Part model, mm, in its own coordinate system. Face numbers are marked on the shaded views. Round coordinates to 2 decimals unless told otherwise and drop trailing zeros. Loops run counter-clockwise (first coordinate to the right, second up) from the corner with the lowest first, then second, coordinate; pieces in that order, holes last. Notation, with made-up numbers: (84, 74) - (104, 74) arc R30 ccw to (104, 109) - close; hole circle Ø4 at (-35.75, 9). An arc over 180 degrees is marked (long way). Put each result on its own line as item: value.
from build123d import *

# Parameters (mm, degrees)
SKETCH1_R               = 9
SKETCH1_R_2             = 8.75
BOSS_EXTRUDE1_DEPTH     = 125
SKETCH2_R               = 2
CUT_EXTRUDE1_DEPTH      = 10
CUT_EXTRUDE1_DEPTH_BACK = 10


with BuildPart() as part:
    # Sketch1 → Boss-Extrude1 (new body)
    with BuildSketch(Plane(origin=(0, 0, 0), x_dir=(1, 0, 0), z_dir=(0, 1, 0))):
        Circle(SKETCH1_R)
        Circle(SKETCH1_R_2, mode=Mode.SUBTRACT)
    extrude(amount=BOSS_EXTRUDE1_DEPTH)

    # Sketch2 → Cut-Extrude1 (cut, two sides)
    with BuildSketch(Plane.XY) as cut_extrude1_sk:
        with Locations((0, 95)):
            Circle(SKETCH2_R)
        with Locations((0, 115)):
            Circle(SKETCH2_R)
        with Locations((0, 10)):
            Circle(SKETCH2_R)
    extrude(amount=CUT_EXTRUDE1_DEPTH, mode=Mode.SUBTRACT)
    extrude(cut_extrude1_sk.sketch, amount=-CUT_EXTRUDE1_DEPTH_BACK, mode=Mode.SUBTRACT)


solid = part.part
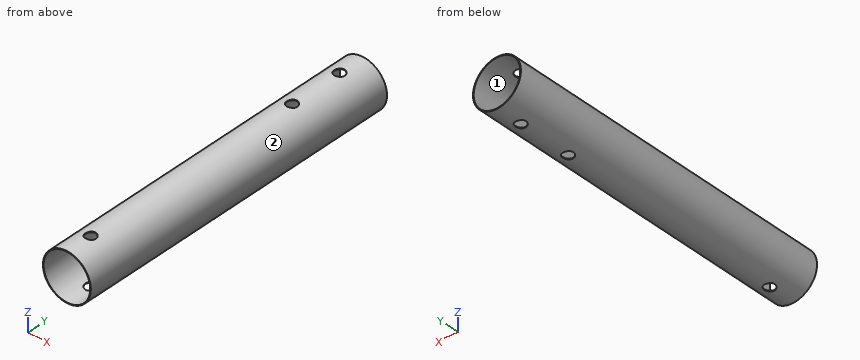
1. Band-saw the part on D-D (y = 73.5). List the corners of the cut face in (x, z).
A:
outline: circle Ø18 at (0, 0); hole circle Ø17.5 at (0, 0)
2. Two-plate mould, pull along Z, no slides. Class the marked faces 1 and 2: pulls with the +Z half, pulls with the -Z half, needs draft (parallel to the pull), parting line crosses it, or undercut.
A:
face 1: undercut
face 2: parting line crosses it
3. Band-saw the part on A-A (x = 0). Give the number of separate pieces and of enclosed holes in the cut face, plus the area to 3 significant figures.
A:
separate pieces: 8
enclosed holes: 0
area: 56.5 mm²
4. Band-saw the part on C-C (y = 115). List the corners of the cut face in (x, z).
A:
outline: (-2, -8.77) - (-2, -8.52) arc R8.75 cw to (-2, 8.52) - (-2, 8.77) arc R9 ccw to start; (2, -8.77) arc R9 ccw to (2, 8.77) - (2, 8.52) arc R8.75 cw to (2, -8.52) - close
5. Probe line 1 along Y through (x, z) = (0, -8.8); line 2 along Z through (x, y) = (0.5, 89); line 3 along X through (y, z) = (23, 6). List the from-to ranges inside material, lowest first. Write a range as [from, to].
A:
line 1: y = [0, 8], [12, 93], [97, 113], [117, 125]
line 2: z = [-8.99, -8.74], [8.74, 8.99]
line 3: x = [-6.71, -6.37], [6.37, 6.71]
6. Pin check, flat tips, straight feed: P1, Ø8, axis at x = 6.5, y = 36, coming from the -Z side; P2, Ø1.5, axis at x = -0.5, y = 78, coming from the -Z side; P3, Ø4, axis at x = 5.5, y = 98.5, coming from the -Z side; P4, Ø1.5, axis at x = -3, y = 79, coming from the -Z side. Stop position of each tip, or through.
A:
P1: stops at z = -8.65
P2: stops at z = -9
P3: stops at z = -8.29
P4: stops at z = -8.71
7. Band-saw the part on B-B (z = 0). List the corners of the cut face in (x, y), plus the area to 3 significant figures.
A:
outline: (-9, 0) - (-8.75, 0) - (-8.75, 125) - (-9, 125) - close; (8.75, 0) - (9, 0) - (9, 125) - (8.75, 125) - close
area: 62.5 mm²
